```python
from build123d import *

# Parameters (mm, degrees)
F0_R     = 3.75
F1_DEPTH = 6.1
F2_W     = 34.5066441072
F2_H     = 13.1774456962
F3_DEPTH = 11
F4_R     = 5.4411545269
F5_R     = 1.5025340948
F6_R     = 2
F7_DEPTH = 4
F8_R     = 3.3571489319


with BuildPart() as f1:
    # F0 (on Top) → F1 (new body)
    with BuildSketch(Plane.XY):
        Polygon((71.75, 4.5), (0, 7.25), (-71.75, 4.5), (-71.75, -4.5), (0, -7.25), (71.75, -4.5), align=None)
        with Locations((-40.375, 0)):
            Circle(F0_R, mode=Mode.SUBTRACT)
        with Locations((40.375, 0)):
            Circle(F0_R, mode=Mode.SUBTRACT)
    extrude(amount=F1_DEPTH)

    # F2 (on face) → F3 (join)
    with BuildSketch(Plane.XY.offset(6.1)):
        Rectangle(F2_W, F2_H)
    extrude(amount=F3_DEPTH)

    # F4
    f4_edges = [f1.edges().sort_by_distance(p)[0] for p in [
        (-17.253322, -6.588723, 11.6),
        (-17.253322, 6.588723, 11.6),
        (17.253322, -6.588723, 11.6),
        (17.253322, 6.588723, 11.6),
    ]]
    fillet(f4_edges, radius=F4_R)

    # F5
    f5_edges = [f1.edges().sort_by_distance(p)[0] for p in [
        (0, 6.588723, 17.1),
        (15.659645, 4.995046, 17.1),
        (17.253322, 0, 17.1),
        (15.659645, -4.995046, 17.1),
        (0, -6.588723, 17.1),
        (-15.659645, -4.995046, 17.1),
        (-17.253322, 0, 17.1),
        (-15.659645, 4.995046, 17.1),
    ]]
    fillet(f5_edges, radius=F5_R)

    # F6 (on face) → F7 (cut)
    with BuildSketch(Plane(origin=(0, 0, 0), x_dir=(1, 0, 0), z_dir=(0, 0, -1))):
        with Locations((-63.125, 0)):
            Circle(F6_R)
        with Locations((63.125, 0)):
            Circle(F6_R)
    extrude(amount=-F7_DEPTH, mode=Mode.SUBTRACT)

    # F8
    f8_edges = [f1.edges().sort_by_distance(p)[0] for p in [
        (71.75, 4.5, 3.05),
        (71.75, -4.5, 3.05),
        (-71.75, 4.5, 3.05),
        (-71.75, -4.5, 3.05),
    ]]
    fillet(f8_edges, radius=F8_R)


solid = f1.part
```
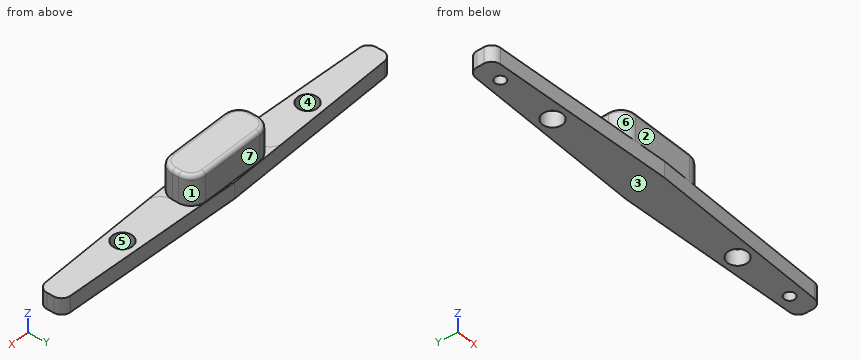
The listing builds one solid part. Answer for the finished solid, in the listing's coordinates (mm). Face numbers are marked on the shaded views. A direction names the side the tool comes from. Round coordinates to 2 decimals unless told otherwise and drop trailing zeros. Loops run counter-clockwise (first coordinate to the right, second up) from the corner with the lowest first, then second, coordinate; pieces in that order, holes last. Notation, with made-up numbers: (77, 7.25) - (126, 7.25) arc R26 cw to (126, 27.25) - close; hole circle Ø1 at (83, 43). An arc over 180 degrees is marked (long way). Return JSON: item names as keys, results as strings. Group by question number.
1. The part is cut by section D-D on x = -38. Determine the outline of the cut face in (y, z), then the cut area to 3 significant figures.
2. The part is cut by section C-C on x = 3.5. Determine the outline of the cut face in (y, z).
3. Consider probe 1 along X at (y, z) = (-2.5, 4.25); probe 2 along Y at (x, z) = (23, 3.25); probe 3 along Y at (x, z) = (-9.5, 11.5). Determine where each line is inside the solid, lowest interval first.
4. Which of the six approach directions +Z, -Z, +X, -X, +Y, -Y give full straight-line access (tool end or side, diameter ignored) to the marked faces 1, 2 and 3?
5. Each of these flat-tipped pins is pushed along its axis until it touches: P1, Ø6, axis at x = -39, z = 1.5, coming from the -Y side; P2, Ø1.8, axis at y = 0, z = 10.5, coming from the -X side; P3, Ø4.5, axis at x = 5, z = 9, coming from the +Y side. Where does it stop, or does it pass through?
6. The part is cut by section A-A on x = 41.5. Determine the outline of the cut face in (y, z).
7. The mould has two halves that part along Y. Classify the marked faces 4, 5, 6 and 7: pulls with the +Y half, pulls with the -Y half, needs draft (parallel to the pull), parting line crosses it, or undercut.
8. The part is cut by section B-B on z = 12.5. Determine the outline of the cut face in (x, y), then the cut area to 3 significant figures.
Resolved:
{
 "1": {"outline": "(-5.79, 0) - (-2.9, 0) - (-2.9, 6.1) - (-5.79, 6.1) - close; (2.9, 0) - (5.79, 0) - (5.79, 6.1) - (2.9, 6.1) - close", "area": "35.3 mm²"},
 "2": {"outline": "(-7.12, 0) - (7.12, 0) - (7.12, 6.1) - (6.59, 6.1) - (6.59, 15.6) arc R1.5 ccw to (5.09, 17.1) - (-5.09, 17.1) arc R1.5 ccw to (-6.59, 15.6) - (-6.59, 6.1) - (-7.12, 6.1) - close"},
 "3": {"probe 1": "x = -71.52 to -43.17, -37.58 to 37.58, 43.17 to 71.52", "probe 2": "y = -6.37 to 6.37", "probe 3": "y = -6.59 to 6.59"},
 "4": {"face 1": "+Z, +X, +Y", "face 2": "+Z, +X, -X, -Y", "face 3": "-Z, +X, -X, +Y, -Y"},
 "5": {"P1": "stops at y = -5.87", "P2": "stops at x = -17.25", "P3": "stops at y = 6.59"},
 "6": {"outline": "(-5.66, 0) - (-3.58, 0) - (-3.58, 6.1) - (-5.66, 6.1) - close; (3.58, 0) - (5.66, 0) - (5.66, 6.1) - (3.58, 6.1) - close"},
 "7": {"face 4": "undercut", "face 5": "undercut", "face 6": "pulls with the -Y half", "face 7": "pulls with the +Y half"},
 "8": {"outline": "(-17.25, -1.15) arc R5.44 ccw to (-11.81, -6.59) - (11.81, -6.59) arc R5.44 ccw to (17.25, -1.15) - (17.25, 1.15) arc R5.44 ccw to (11.81, 6.59) - (-11.81, 6.59) arc R5.44 ccw to (-17.25, 1.15) - close", "area": "429 mm²"}
}
